Geometry: see drawing. Coordinates: mm, zero at the bounding-box minimum. Round coordinates to 2 decimals unless told otherwise and drop trailing zeros. Loops run counter-clockwise (first coordinate to the right, second up) from the corner with the lowest first, then second, coordinate; pieces in that order, holes last. Notation, with made-up numbers: (20, 86.25) - (73, 86.25) arc R10 cw to (73, 99.25) - close; hole circle Ø6 at (60, 76). An arc over 180 degrees is marked (long way). One line per question, with ' | ' between items. Start each with the question number.
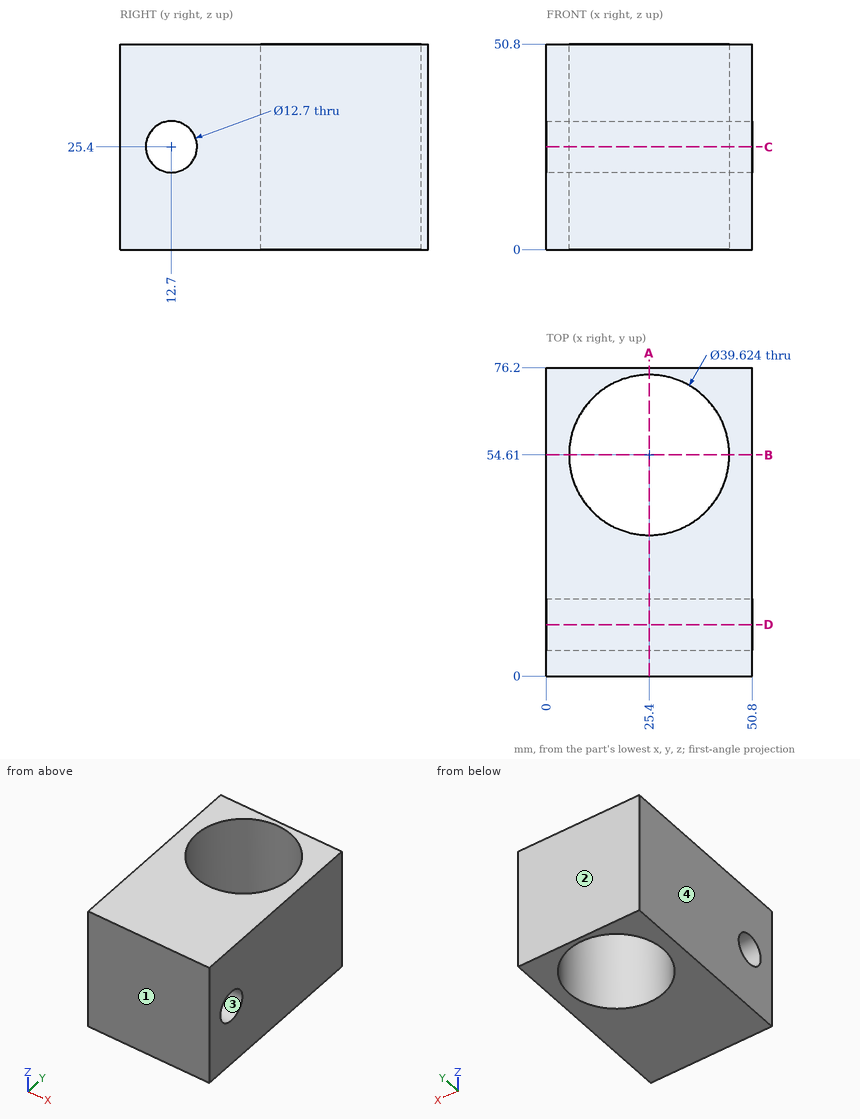
(1) Section D-D, the plane y = 12.7. Output: boundary loops of the cut face in (x, z).
(2) Pull-direction query (Y, two-part tool) for the marked faces 1, 2, 3 and 4; classes: released by +Y, released by -Y, zero draft, split by the parting line, or undercut.
(3) Section C-C, the plane z = 25.4. Output: boundary loops of the cut face in (x, y), plus the area to 3 significant figures.
(4) Section A-A, the plane x = 25.4. Output: boundary loops of the cut face in (y, z).
(5) Section B-B, the plane y = 54.61. Output: boundary loops of the cut face in (x, z), plus the area to 3 significant figures.
(6) Line query: line 1 along X through (y, z) = (54, 25); line 2 along Y through (x, z) = (25, 25); line 3 along Y through (x, z) = (25, 14). Output: solid intervals per line, ascending. Write a range as from..to.
Derived:
1) outline: (0, 0) - (50.8, 0) - (50.8, 19.05) - (0, 19.05) - close; (0, 31.75) - (50.8, 31.75) - (50.8, 50.8) - (0, 50.8) - close
2) face 1: released by -Y | face 2: released by +Y | face 3: undercut | face 4: zero draft
3) outline: (0, 0) - (50.8, 0) - (50.8, 6.35) - (0, 6.35) - close; (0, 19.05) - (50.8, 19.05) - (50.8, 76.2) - (0, 76.2) - close; hole circle Ø39.62 at (25.4, 54.61) | area: 1,990 mm²
4) outline: (0, 0) - (34.8, 0) - (34.8, 50.8) - (0, 50.8) - close; (74.42, 0) - (76.2, 0) - (76.2, 50.8) - (74.42, 50.8) - close; hole circle Ø12.7 at (12.7, 25.4)
5) outline: (0, 0) - (5.59, 0) - (5.59, 50.8) - (0, 50.8) - close; (45.21, 0) - (50.8, 0) - (50.8, 50.8) - (45.21, 50.8) - close | area: 568 mm²
6) line 1: x = 0..5.6, 45.2..50.8 | line 2: y = 0..6.36, 19.04..34.8, 74.42..76.2 | line 3: y = 0..34.8, 74.42..76.2
